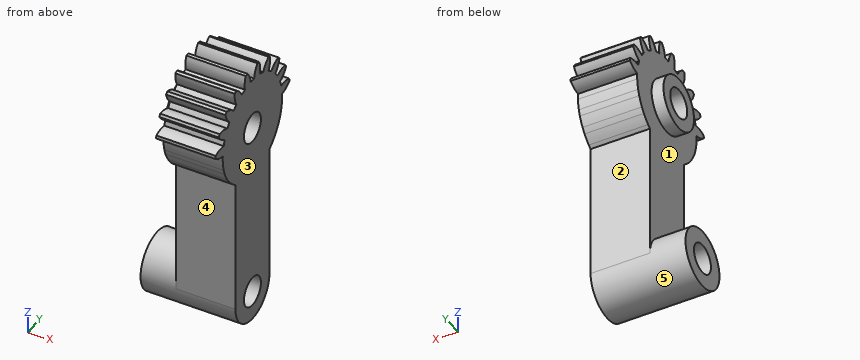
```python
from build123d import *

# Parameters (mm, degrees)
SKETCH1_R           = 2.5
BOSS_EXTRUDE1_DEPTH = 10
SKETCH2_R           = 2.5
BOSS_EXTRUDE2_DEPTH = 10
SKETCH3_R           = 5
SKETCH3_R_2         = 2.5
BOSS_EXTRUDE3_DEPTH = 6
SKETCH4_R           = 2.5
CUT_EXTRUDE1_DEPTH  = 5
SKETCH6_R           = 1.5
CUT_EXTRUDE2_DEPTH  = 40.400672482
CUT_EXTRUDE3_START  = -3
SKETCH7_R           = 2.5
CUT_EXTRUDE3_DEPTH  = 3
SKETCH8_R           = 4.5
SKETCH8_R_2         = 2.5
BOSS_EXTRUDE4_DEPTH = 2
CUT_EXTRUDE4_DEPTH  = 42.078132772


with BuildPart() as part:
    # Sketch1 → Boss-Extrude1 (new body)
    with BuildSketch(Plane(origin=(4.043870029, 0, 0), x_dir=(0, 0, -1), z_dir=(1, 0, 0))):
        with BuildLine():
            ThreePointArc((-10.029541992, 0.342879069), (-9.019080639, -0.304016541), (-7.862233613, -0.622153359))
            ThreePointArc((-7.862233613, -0.622153359), (-7.876528296, -1.122077366), (-7.862233613, -1.622001374))
            ThreePointArc((-7.862233613, -1.622001374), (-9.019080639, -1.940138191), (-10.029541992, -2.587033801))
            ThreePointArc((-10.029541992, -2.587033801), (-9.992100042, -2.842856482), (-9.948655897, -3.097728508))
            ThreePointArc((-9.948655897, -3.097728508), (-8.787748306, -3.400713063), (-7.58921172, -3.345793765))
            ThreePointArc((-7.58921172, -3.345793765), (-7.448321757, -3.82566705), (-7.280241692, -4.296705735))
            ThreePointArc((-7.280241692, -4.296705735), (-8.282158911, -4.956757219), (-9.043263028, -5.884241235))
            ThreePointArc((-9.043263028, -5.884241235), (-8.928600062, -6.115972863), (-8.808522437, -6.344945585))
            ThreePointArc((-8.808522437, -6.344945585), (-7.610806331, -6.274360846), (-6.487901298, -5.851761317))
            ThreePointArc((-6.487901298, -5.851761317), (-6.20561798, -6.264610538), (-5.90020538, -6.660655353))
            ThreePointArc((-5.90020538, -6.660655353), (-6.649118154, -7.598011066), (-7.086362862, -8.715294889))
            ThreePointArc((-7.086362862, -8.715294889), (-6.905702889, -8.900251959), (-6.720745819, -9.080911932))
            ThreePointArc((-6.720745819, -9.080911932), (-5.603461996, -8.643667224), (-4.666106283, -7.89475445))
            ThreePointArc((-4.666106283, -7.89475445), (-4.270061468, -8.20016705), (-3.857212247, -8.482450368))
            ThreePointArc((-3.857212247, -8.482450368), (-4.279811776, -9.605355401), (-4.350396515, -10.803071507))
            ThreePointArc((-4.350396515, -10.803071507), (-4.121423793, -10.923149132), (-3.889692165, -11.037812099))
            ThreePointArc((-3.889692165, -11.037812099), (-2.962208149, -10.276707981), (-2.302156665, -9.274790762))
            ThreePointArc((-2.302156665, -9.274790762), (-1.83111798, -9.442870827), (-1.351244695, -9.583760791))
            ThreePointArc((-1.351244695, -9.583760791), (-1.406163992, -10.782297376), (-1.103179437, -11.943204968))
            ThreePointArc((-1.103179437, -11.943204968), (-0.848307411, -11.986649113), (-0.592484731, -12.024091063))
            ThreePointArc((-0.592484731, -12.024091063), (0.054410879, -11.01362971), (0.372547697, -9.856782684))
            ThreePointArc((0.372547697, -9.856782684), (0.872471704, -9.871077366), (1.372395712, -9.856782684))
            ThreePointArc((1.372395712, -9.856782684), (1.690532529, -11.01362971), (2.337428139, -12.024091063))
            ThreePointArc((2.337428139, -12.024091063), (2.59325082, -11.986649113), (2.848122846, -11.943204968))
            ThreePointArc((2.848122846, -11.943204968), (3.151107401, -10.782297376), (3.096188103, -9.583760791))
            ThreePointArc((3.096188103, -9.583760791), (3.576061388, -9.442870827), (4.047100073, -9.274790762))
            ThreePointArc((4.047100073, -9.274790762), (4.707151558, -10.276707981), (5.634635573, -11.037812099))
            ThreePointArc((5.634635573, -11.037812099), (5.866367201, -10.923149132), (6.095339923, -10.803071507))
            ThreePointArc((6.095339923, -10.803071507), (6.024755184, -9.605355401), (5.602155655, -8.482450368))
            ThreePointArc((5.602155655, -8.482450368), (6.015004877, -8.20016705), (6.411049691, -7.89475445))
            ThreePointArc((6.411049691, -7.89475445), (7.348405404, -8.643667224), (8.465689227, -9.080911932))
            ThreePointArc((8.465689227, -9.080911932), (8.650646297, -8.900251959), (8.83130627, -8.715294889))
            ThreePointArc((8.83130627, -8.715294889), (8.394061563, -7.598011066), (7.645148788, -6.660655353))
            ThreePointArc((7.645148788, -6.660655353), (7.950561388, -6.264610538), (8.232844706, -5.851761317))
            ThreePointArc((8.232844706, -5.851761317), (9.355749739, -6.274360846), (10.553465846, -6.344945585))
            ThreePointArc((10.553465846, -6.344945585), (10.67354347, -6.115972863), (10.788206437, -5.884241235))
            ThreePointArc((10.788206437, -5.884241235), (10.02710232, -4.956757219), (9.0251851, -4.296705735))
            ThreePointArc((9.0251851, -4.296705735), (9.193265165, -3.82566705), (9.334155129, -3.345793765))
            ThreePointArc((9.334155129, -3.345793765), (10.532691714, -3.400713063), (11.693599306, -3.097728508))
            ThreePointArc((11.693599306, -3.097728508), (11.737043451, -2.842856482), (11.774485401, -2.587033801))
            ThreePointArc((11.774485401, -2.587033801), (10.764024048, -1.940138191), (9.607177022, -1.622001374))
            ThreePointArc((9.607177022, -1.622001374), (9.621471704, -1.122077366), (9.607177022, -0.622153359))
            ThreePointArc((9.607177022, -0.622153359), (10.764024048, -0.304016541), (11.774485401, 0.342879069))
            ThreePointArc((11.774485401, 0.342879069), (11.737043451, 0.598701749), (11.693599306, 0.853573775))
            ThreePointArc((11.693599306, 0.853573775), (10.532691714, 1.156558331), (9.334155129, 1.101639033))
            ThreePointArc((9.334155129, 1.101639033), (9.193265165, 1.581512318), (9.0251851, 2.052551003))
            ThreePointArc((9.0251851, 2.052551003), (10.02710232, 2.712602487), (10.788206437, 3.640086503))
            ThreePointArc((10.788206437, 3.640086503), (10.67354347, 3.871818131), (10.553465846, 4.100790853))
            ThreePointArc((10.553465846, 4.100790853), (9.355749739, 4.030206114), (8.232844706, 3.607606585))
            ThreePointArc((8.232844706, 3.607606585), (7.950561388, 4.020455806), (7.645148788, 4.416500621))
            ThreePointArc((7.645148788, 4.416500621), (8.394061563, 5.353856334), (8.83130627, 6.471140157))
            ThreePointArc((8.83130627, 6.471140157), (8.650646297, 6.656097227), (8.465689227, 6.8367572))
            ThreePointArc((8.465689227, 6.8367572), (7.348405404, 6.399512492), (6.411049691, 5.650599718))
            ThreePointArc((6.411049691, 5.650599718), (6.015004877, 5.956012318), (5.602155655, 6.238295636))
            ThreePointArc((5.602155655, 6.238295636), (6.024755184, 7.361200669), (6.095339923, 8.558916775))
            ThreePointArc((6.095339923, 8.558916775), (5.866367201, 8.6789944), (5.634635573, 8.793657366))
            ThreePointArc((5.634635573, 8.793657366), (4.707151558, 8.032553249), (4.047100073, 7.03063603))
            ThreePointArc((4.047100073, 7.03063603), (3.576061388, 7.198716095), (3.096188103, 7.339606058))
            ThreePointArc((3.096188103, 7.339606058), (3.151107401, 8.538142644), (2.848122846, 9.699050235))
            ThreePointArc((2.848122846, 9.699050235), (2.59325082, 9.74249438), (2.337428139, 9.779936331))
            ThreePointArc((2.337428139, 9.779936331), (1.690532529, 8.769474978), (1.372395712, 7.612627952))
            ThreePointArc((1.372395712, 7.612627952), (0.872471704, 7.626922634), (0.372547697, 7.612627952))
            ThreePointArc((0.372547697, 7.612627952), (0.054410879, 8.769474978), (-0.592484731, 9.779936331))
            ThreePointArc((-0.592484731, 9.779936331), (-0.848307411, 9.74249438), (-1.103179437, 9.699050235))
            ThreePointArc((-1.103179437, 9.699050235), (-1.406163992, 8.538142644), (-1.351244695, 7.339606058))
            ThreePointArc((-1.351244695, 7.339606058), (-1.83111798, 7.198716095), (-2.302156665, 7.03063603))
            ThreePointArc((-2.302156665, 7.03063603), (-2.962208149, 8.032553249), (-3.889692165, 8.793657366))
            ThreePointArc((-3.889692165, 8.793657366), (-4.121423793, 8.6789944), (-4.350396515, 8.558916775))
            ThreePointArc((-4.350396515, 8.558916775), (-4.279811776, 7.361200669), (-3.857212247, 6.238295636))
            ThreePointArc((-3.857212247, 6.238295636), (-4.270061468, 5.956012318), (-4.666106283, 5.650599718))
            ThreePointArc((-4.666106283, 5.650599718), (-5.603461996, 6.399512492), (-6.720745819, 6.8367572))
            ThreePointArc((-6.720745819, 6.8367572), (-6.905702889, 6.656097227), (-7.086362862, 6.471140157))
            ThreePointArc((-7.086362862, 6.471140157), (-6.649118154, 5.353856334), (-5.90020538, 4.416500621))
            ThreePointArc((-5.90020538, 4.416500621), (-6.20561798, 4.020455806), (-6.487901298, 3.607606585))
            ThreePointArc((-6.487901298, 3.607606585), (-7.610806331, 4.030206114), (-8.808522437, 4.100790853))
            ThreePointArc((-8.808522437, 4.100790853), (-8.928600062, 3.871818131), (-9.043263028, 3.640086503))
            ThreePointArc((-9.043263028, 3.640086503), (-8.282158911, 2.712602487), (-7.280241692, 2.052551003))
            ThreePointArc((-7.280241692, 2.052551003), (-7.448321757, 1.581512318), (-7.58921172, 1.101639033))
            ThreePointArc((-7.58921172, 1.101639033), (-8.787748306, 1.156558331), (-9.948655897, 0.853573775))
            ThreePointArc((-9.948655897, 0.853573775), (-9.992100042, 0.598701749), (-10.029541992, 0.342879069))
        make_face()
        with Locations(Location((0.872471704, -1.122077366, 0), (0, 0, 180))):
            Circle(SKETCH1_R, mode=Mode.SUBTRACT)
    extrude(amount=-BOSS_EXTRUDE1_DEPTH)

    # Sketch2 → Boss-Extrude2 (add)
    with BuildSketch(Plane(origin=(4.043870029, 0, 0), x_dir=(0, 0, -1), z_dir=(1, 0, 0))):
        with BuildLine():
            Line((0.872471704, 3.877922634), (30.872471704, 3.877922634))
            ThreePointArc((30.872471704, 3.877922634), (35.872471704, -1.122077366), (30.872471704, -6.122077366))
            Line((30.872471704, -6.122077366), (0.872471704, -6.122077366))
            ThreePointArc((0.872471704, -6.122077366), (-4.127528296, -1.122077366), (0.872471704, 3.877922634))
        make_face()
        with Locations((30.872471704, -1.122077366)):
            Circle(SKETCH2_R, mode=Mode.SUBTRACT)
    extrude(amount=-BOSS_EXTRUDE2_DEPTH)

    # Sketch3 → Boss-Extrude3 (add)
    with BuildSketch(Plane.ZY.offset(5.956129971)):
        with Locations(Location((-30.872471704, -1.122077366, 0), (0, 0, 270))):
            Circle(SKETCH3_R)
        with Locations(Location((-30.872471704, -1.122077366, 0), (0, 0, 180))):
            Circle(SKETCH3_R_2, mode=Mode.SUBTRACT)
    extrude(amount=BOSS_EXTRUDE3_DEPTH)

    # Sketch4 → Cut-Extrude1 (cut)
    with BuildSketch(Plane(origin=(4.043870029, 0, 0), x_dir=(0, 0, -1), z_dir=(1, 0, 0))):
        with Locations((0.872471704, -1.122077366)):
            Circle(SKETCH4_R)
    extrude(amount=-CUT_EXTRUDE1_DEPTH, mode=Mode.SUBTRACT)

    # Sketch6 → Cut-Extrude2 (cut, through all)
    with BuildSketch(Plane(origin=(-0.956129971, 0, 0), x_dir=(0, 0, -1), z_dir=(1, 0, 0))):
        with Locations((0.872471704, -1.122077366)):
            Circle(SKETCH6_R)
    extrude(amount=-CUT_EXTRUDE2_DEPTH, mode=Mode.SUBTRACT)

    # Sketch7 → Cut-Extrude3 (cut)
    with BuildSketch(Plane.ZY.offset(5.956129971).offset(CUT_EXTRUDE3_START)):
        with Locations(Location((-0.872471704, -1.122077366, 0), (0, 0, 180))):
            Circle(SKETCH7_R)
    extrude(amount=CUT_EXTRUDE3_DEPTH, mode=Mode.SUBTRACT)

    # Sketch8 → Boss-Extrude4 (add)
    with BuildSketch(Plane.ZY.offset(5.956129971)):
        with Locations(Location((-0.872471704, -1.122077366, 0), (0, 0, 180))):
            Circle(SKETCH8_R)
        with Locations(Location((-0.872471704, -1.122077366, 0), (0, 0, 180))):
            Circle(SKETCH8_R_2, mode=Mode.SUBTRACT)
    extrude(amount=BOSS_EXTRUDE4_DEPTH)

    # Sketch9 → Cut-Extrude4 (cut, through all)
    with BuildSketch(Plane(origin=(4.043870029, 0, 0), x_dir=(0, 0, -1), z_dir=(1, 0, 0))):
        with BuildLine():
            Line((11.302349515, -6.122077366), (8.051956435, -6.122077366))
            ThreePointArc((8.051956435, -6.122077366), (4.922163112, -8.877398152), (0.872471704, -9.871077366))
            Line((0.872471704, -9.871077366), (0.872471704, -12.68850945))
            ThreePointArc((0.872471704, -12.68850945), (7.034865343, -10.910195458), (11.302349515, -6.122077366))
        make_face()
        with BuildLine():
            Line((11.302349515, 3.877922634), (8.051956435, 3.877922634))
            ThreePointArc((8.051956435, 3.877922634), (4.922163112, 6.63324342), (0.872471704, 7.626922634))
            Line((0.872471704, 7.626922634), (0.872471704, 10.444354718))
            ThreePointArc((0.872471704, 10.444354718), (7.034865343, 8.666040726), (11.302349515, 3.877922634))
        make_face()
    extrude(amount=-CUT_EXTRUDE4_DEPTH, mode=Mode.SUBTRACT)


solid = part.part
```
Source: CAD feature listing. Evaluate the final solid. Frame: model axes, mm. Face numbers are marked on the shaded views. A direction names the side the tool comes from. Round coordinates to 2 decimals unless told otherwise and drop trailing zeros. Order: outer loops, then holes, each group sorted by start corner. A loop starts at its lowest first (then second) coordinate and runs counter-clockwise, first axis right, second up. Notation, with made-up numbers: (4, 15.25) -> (11, 15.25) arc R20 ccw to (11, 21.25) -> close; hole circle Ø4 at (52.5, -33.75). An arc over 180 degrees is marked (long way). Use CSV: the item, a comma, the result in double quotes.
(1) Ray query, L1, parallel to X at y = 0.25, z = 0.5; L2, parallel to X at y = -4, z = -22; L3, parallel to Y at x = -3, z = -3. Return the intervals inside material, ascending.
Report:
L1,"-2.96 to -0.96"
L2,"-5.96 to 4.04"
L3,"-9.61 to -2.43, 0.19 to 7.36"
(2) Section A-A on x = -6.5. Return the cut outline in (y, z).
Report:
outline,"circle Ø10 at (-1.12, -30.87); circle Ø9 at (-1.12, -0.87); hole circle Ø5 at (-1.12, -30.87); hole circle Ø5 at (-1.12, -0.87)"
(3) Access query for the marked faces 3, 4 and 5. Directions: +Z, -Z, +X, -X, +Y, -Y. A direction counts if a zero-diameter tool reaches every point of the face in a straight line with its end or side. Return the directions, or none.
Report:
face 3,"+Z, -Z, +X, +Y, -Y"
face 4,"-Z, +X, -X, -Y"
face 5,"-X"
(4) Section B-B on z = -9.5. Return the cut outline in (x, y), and give its area (3 significant figures).
Report:
outline,"(-5.96, -6.12) -> (4.04, -6.12) -> (4.04, 3.88) -> (-5.96, 3.88) -> close"
area,"100 mm^2"
(5) First-contact query: pin 1 Ø6 at (y, z) = (1.5, -23) entering from -X; pin 2 Ø3 at (x, y) = (-5.5, -8) entering from -Z; pin 3 Ø3 at (x, z) = (-4.5, -27.5) entering from -Y. Flat tips, straight axial feed; report the tip coordinate or a pass-through.
Report:
pin 1,"x = -5.96"
pin 2,"z = -7.77"
pin 3,"y = -6.12"
(6) Section C-C on y = -7.25. Return the cut outline in (x, z), and give its area (3 significant figures).
Report:
outline,"(-5.96, -7.12) -> (4.04, -7.12) -> (4.04, 6.42) -> (-5.96, 6.42) -> close"
area,"135 mm^2"
(7) Section D-D on x = -0.25. Count the separate pieces of the cut face and the enclosed holes in it, and give its area (3 significant figures).
Report:
separate pieces,"1"
enclosed holes,"2"
area,"489 mm^2"
(8) Pull-direction query (Z, two-part tool) for the marked faces 1 and 2; classes: +Z half, -Z half, draft (parallel to the pull), parting line (faces both ways), or undercut.
Report:
face 1,"undercut"
face 2,"draft"
